Read the model definition and answer for the solid it produces. Units are mm, in the model's axes. A direction names the side the tool comes from. Coordinates: 2 decimals unless noted, no trailing zeros. Write each loop counter-clockwise with the first axis right and the second up, starting at its lowest first coordinate (ties: lowest second). Pieces come first, ordered by that corner, then holes. Notation, with made-up numbers: (17.25, -36) -> (71.25, -36) arc R23 cw to (71.25, 3) -> close; hole circle Ø8 at (14, 6.25). An arc over 180 degrees is marked (long way). One line per item, written item: value. Start each with the question number.
1. Given P1, Ø23.5, axis at x = 0, z = 0, coming from the -Y side; P2, Ø1.5, axis at x = 48.5, y = 52, coming from the -Z side; P3, Ø12, axis at x = -59.5, z = 8, coming from the +Y side; P4, Ø2, axis at y = -19.5, z = -29.5, coming from the -X side, each flat-ended and moving along its own axis, determine where each tip first touches the part or whether it passes through.
2. Find section C-C, the plane z = -65. Write down the section's boundary in (x, y).
3. For a pull along Z with two mould halves and no side action, classify faces 1 (the cylindrical face through (29.136, 1.426, 23.276)), 2 (the cylindrical face through (-11.99, -24.46, -0.53)), 3 (the flat face through (11, -57, -6)), 4 (the flat face through (8, 33, 8)) as pulls with the +Z half, pulls with the -Z half, needs draft (parallel to the pull), parting line crosses it, or undercut.
4. Find section A-A, the plane y = 11.5. Write down the section's boundary in (x, z) (3 decimals).
5. Consider line 1 along Y through (x, z) = (0.5, -42); line 2 along X through (y, z) = (56.5, 1); line 3 along Z through (x, y) = (-3, 3). Determine where each line is inside the solid, lowest interval first.
6. Find section D-D, the plane y = -39.5. Write down the section's boundary in (x, z), and give its area (3 significant figures).
7. For faces 5 (the flat face through (28.572, 39.51, -21.882)), 6 (the cylindrical face through (56, 40, 0)), 7 (the flat face through (-28.572, 39.51, 21.882)), 8 (the flat face through (29.05, 39.51, 21.69)), 9 (the flat face through (8, 45, 8)), determine the directions among +Z, -Z, +X, -X, +Y, -Y from which every point of the face is accessible in a straight line to the end or side of a thin tool.
8. Find section B-B, the plane y = 64.5. Write down the section's boundary in (x, z) (3 decimals), and give its area (3 significant figures).
```python
from build123d import *

# Parameters (mm, degrees)
SKETCH1_R                   = 7.5
SKETCH1_R_2                 = 19.5
SKETCH1_R_3                 = 10.5
BOSS_EXTRUDE1_DEPTH         = 75
SKETCH1_3_R                 = 85.5
SKETCH1_3_R_2               = 7.5
BOSS_EXTRUDE2_DEPTH         = 15
F_1_0MM_DOWEL_HOLE1_D       = 15
F_1_0MM_DOWEL_HOLE1_DEPTH   = 25.493545357
F_1_0MM_DOWEL_HOLE1_TIP     = 4.506454643
SKETCH4_R                   = 42
SKETCH5_R                   = 24
ADVANCEDHOLE1_START         = -57
ADVANCEDHOLE1_OUTLINE_R     = 10.5
ADVANCEDHOLE1_DEPTH         = 132
ADVANCEDHOLE1_START_2       = 45
ADVANCEDHOLE1_2_OUTLINE_R   = 19.5
ADVANCEDHOLE1_2_OUTLINE_R_2 = 10.5
ADVANCEDHOLE1_2_DEPTH       = 30
ADVANCEDHOLE1_START_3       = 9
ADVANCEDHOLE1_3_OUTLINE_R   = 19.5
ADVANCEDHOLE1_3_OUTLINE_R_2 = 10.5
ADVANCEDHOLE1_3_DEPTH       = 24
ADVANCEDHOLE1_4_OUTLINE_R   = 12
ADVANCEDHOLE1_4_OUTLINE_R_2 = 10.5
ADVANCEDHOLE1_4_DEPTH       = 66
FILLET1_R                   = 5


# Read off the part's stored shape, not the designer's step: AdvancedHole1
with BuildPart() as part:
    # Sketch1 → Boss-Extrude1 (new body)
    # profile 1 of 5: a face of its own
    with BuildSketch(Plane(origin=(0, 0, 0), x_dir=(1, 0, 0), z_dir=(0, 1, 0))):
        with BuildLine():
            Line((11.625, 28.737769137), (46, 14.832396974))
            ThreePointArc((46, 14.832396974), (56, 0), (46, -14.832396974))
            Line((46, -14.832396974), (11.625, -28.737769137))
            ThreePointArc((11.625, -28.737769137), (0, -31), (-11.625, -28.737769137))
            Line((-11.625, -28.737769137), (-46, -14.832396974))
            ThreePointArc((-46, -14.832396974), (-56, 0), (-46, 14.832396974))
            Line((-46, 14.832396974), (-11.625, 28.737769137))
            ThreePointArc((-11.625, 28.737769137), (0, 31), (11.625, 28.737769137))
        make_face()
        with Locations((-40, 0)):
            Circle(SKETCH1_R, mode=Mode.SUBTRACT)
        with Locations((40, 0)):
            Circle(SKETCH1_R, mode=Mode.SUBTRACT)
        Circle(SKETCH1_R_2, mode=Mode.SUBTRACT)
    # profile 2 of 5: a face of its own
    with BuildSketch(Plane(origin=(0, 0, 0), x_dir=(1, 0, 0), z_dir=(0, 1, 0))):
        Circle(SKETCH1_R_2)
        Circle(SKETCH1_R_3, mode=Mode.SUBTRACT)
    # profile 3 of 5: a face of its own
    with BuildSketch(Plane(origin=(0, 0, 0), x_dir=(1, 0, 0), z_dir=(0, 1, 0))):
        Circle(SKETCH1_R_3)
    # profile 4 of 5: a face of its own
    with BuildSketch(Plane(origin=(0, 0, 0), x_dir=(1, 0, 0), z_dir=(0, 1, 0))):
        with Locations((40, 0)):
            Circle(SKETCH1_R)
    # profile 5 of 5: a face of its own
    with BuildSketch(Plane(origin=(0, 0, 0), x_dir=(1, 0, 0), z_dir=(0, 1, 0))):
        with Locations((-40, 0)):
            Circle(SKETCH1_R)
    extrude(amount=BOSS_EXTRUDE1_DEPTH)

    # Sketch1<3> → Boss-Extrude2 (add)
    with BuildSketch(Plane(origin=(0, 0, 0), x_dir=(1, 0, 0), z_dir=(0, 1, 0))):
        with Locations(Location((0, 0, 0), (0, 0, 270))):
            Circle(SKETCH1_3_R)
        with Locations(Location((44.547727215, 44.547727215, 0), (0, 0, 270))):
            Circle(SKETCH1_3_R_2, mode=Mode.SUBTRACT)
        with Locations(Location((44.547727215, -44.547727215, 0), (0, 0, 270))):
            Circle(SKETCH1_3_R_2, mode=Mode.SUBTRACT)
        with Locations(Location((-44.547727215, -44.547727215, 0), (0, 0, 270))):
            Circle(SKETCH1_3_R_2, mode=Mode.SUBTRACT)
        with Locations(Location((-44.547727215, 44.547727215, 0), (0, 0, 270))):
            Circle(SKETCH1_3_R_2, mode=Mode.SUBTRACT)
    extrude(amount=-BOSS_EXTRUDE2_DEPTH)

    # Ø1.0mm Dowel Hole1
    with Locations(Plane(origin=(-40, 75, 0), x_dir=(0, 0, 1), z_dir=(0, 1, 0))):
        with Locations((0, 0), (0, 80)):
            Hole(F_1_0MM_DOWEL_HOLE1_D / 2, depth=F_1_0MM_DOWEL_HOLE1_DEPTH)
            with Locations((0, 0, -(F_1_0MM_DOWEL_HOLE1_DEPTH + F_1_0MM_DOWEL_HOLE1_TIP / 2))):  # 118° drill point
                Cone(0, F_1_0MM_DOWEL_HOLE1_D / 2, F_1_0MM_DOWEL_HOLE1_TIP, mode=Mode.SUBTRACT)

    # Sketch4 → Loft1 section 0
    with BuildSketch(Plane.XZ.offset(15)):
        Circle(SKETCH4_R)
    # Sketch5 → Loft1 section 1
    with BuildSketch(Plane(origin=(0, -57, 0), x_dir=(-1, 0, 0), z_dir=(0, -1, 0))):
        Circle(SKETCH5_R)
    loft()

    # AdvancedHole1 outline → AdvancedHole1 (cut)
    with BuildSketch(Plane(origin=(0, 0, 0), x_dir=(1, 0, 0), z_dir=(0, 1, 0)).offset(ADVANCEDHOLE1_START)):
        Circle(ADVANCEDHOLE1_OUTLINE_R)
    extrude(amount=ADVANCEDHOLE1_DEPTH, mode=Mode.SUBTRACT)

    # AdvancedHole1 2 outline → AdvancedHole1 2 (cut)
    with BuildSketch(Plane(origin=(0, 0, 0), x_dir=(1, 0, 0), z_dir=(0, 1, 0)).offset(ADVANCEDHOLE1_START_2)):
        Circle(ADVANCEDHOLE1_2_OUTLINE_R)
        Circle(ADVANCEDHOLE1_2_OUTLINE_R_2, mode=Mode.SUBTRACT)
    extrude(amount=ADVANCEDHOLE1_2_DEPTH, mode=Mode.SUBTRACT)

    # AdvancedHole1 3 outline → AdvancedHole1 3 (cut)
    with BuildSketch(Plane(origin=(0, 0, 0), x_dir=(1, 0, 0), z_dir=(0, 1, 0)).offset(ADVANCEDHOLE1_START_3)):
        Circle(ADVANCEDHOLE1_3_OUTLINE_R)
        Circle(ADVANCEDHOLE1_3_OUTLINE_R_2, mode=Mode.SUBTRACT)
    extrude(amount=ADVANCEDHOLE1_3_DEPTH, mode=Mode.SUBTRACT)

    # AdvancedHole1 4 outline → AdvancedHole1 4 (cut)
    with BuildSketch(Plane(origin=(0, 0, 0), x_dir=(1, 0, 0), z_dir=(0, 1, 0)).offset(ADVANCEDHOLE1_START)):
        Circle(ADVANCEDHOLE1_4_OUTLINE_R)
        Circle(ADVANCEDHOLE1_4_OUTLINE_R_2, mode=Mode.SUBTRACT)
    extrude(amount=ADVANCEDHOLE1_4_DEPTH, mode=Mode.SUBTRACT)

    # Fillet1
    fillet1_edges = [part.edges().sort_by_distance(p)[0] for p in [
        (28.8125, 0, 21.785083056),
        (0, 0, 31),
        (-28.8125, 0, 21.785083056),
        (-56, 0, 0),
        (-28.8125, 0, -21.785083056),
        (0, 0, -31),
        (28.8125, 0, -21.785083056),
        (56, 0, 0),
    ]]
    fillet(fillet1_edges, radius=FILLET1_R)


solid = part.part
```
Answer block:
1. P1: stops at y = 33
1. P2: stops at z = -14
1. P3: stops at y = 75
1. P4: stops at x = -28.34
2. outline: (-55.55, -15) -> (55.55, -15) -> (55.55, 0) -> (-55.55, 0) -> close
3. face 1: pulls with the +Z half
3. face 2: undercut
3. face 3: needs draft
3. face 4: undercut
4. outline: (-46, -14.832) -> (-11.625, -28.738) arc R31 ccw to (11.625, -28.738) -> (46, -14.832) arc R16 ccw to (46, 14.832) -> (11.625, 28.738) arc R31 ccw to (-11.625, 28.738) -> (-46, 14.832) arc R16 ccw to start; hole circle Ø39 at (0, 0)
5. line 1: y = -15 to 0
5. line 2: x = -55.97 to -47.43, -32.57 to -19.47, 19.47 to 32.57, 47.43 to 55.97
5. line 3: z = -31.27 to -11.62, 11.62 to 31.27
6. outline: circle Ø63 at (0, 0); hole circle Ø24 at (0, 0)
6. area: 2,660 mm2
7. face 5: -Z, +X, +Y
7. face 6: +X, +Y
7. face 7: +Z, -X, +Y
7. face 8: +Z, +X, +Y
7. face 9: +Y
8. outline: (-46, -14.832) -> (-11.625, -28.738) arc R31 ccw to (11.625, -28.738) -> (46, -14.832) arc R16 ccw to (46, 14.832) -> (11.625, 28.738) arc R31 ccw to (-11.625, 28.738) -> (-46, 14.832) arc R16 ccw to start; hole circle Ø15 at (-40, 0); hole circle Ø39 at (0, 0); hole circle Ø15 at (40, 0)
8. area: 3,280 mm2
